The listing builds one solid part. Answer for the finished solid, in the listing's coordinates (mm). Face numbers are marked on the shaded views. A direction names the side the tool comes from. Give positions to 0.01 mm unless a question says otherwise; leave off trailing zeros. Write each loop counter-clockwise with the first axis right and the second up, starting at its lowest first coordinate (ties: lowest second). Pieces come first, ordered by that corner, then holes.
```python
from build123d import *

# Parameters (mm, degrees)
SKETCH1_W           = 122.77
SKETCH1_H           = 93
SKETCH1_R           = 1.63
BOSS_EXTRUDE1_DEPTH = 2
SKETCH2_W           = 2
SKETCH2_H           = 93
BOSS_EXTRUDE2_DEPTH = 31
SKETCH3_W           = 28.885
SKETCH3_H           = 73
SKETCH3_W_2         = 21
SKETCH3_H_2         = 83
CUT_EXTRUDE1_DEPTH  = 176.967075005


with BuildPart() as part:
    # Sketch1 → Boss-Extrude1 (new body)
    with BuildSketch(Plane(origin=(0, 0, 0), x_dir=(1, 0, 0), z_dir=(0, 1, 0))):
        with Locations((-105.371378726, 0.358527933)):
            Rectangle(SKETCH1_W, SKETCH1_H)
        with Locations(Location((-161.756378726, 41.858527933, 0), (0, 0, 270))):
            Circle(SKETCH1_R, mode=Mode.SUBTRACT)
        with Locations(Location((-48.986378726, 41.858527933, 0), (0, 0, 270))):
            Circle(SKETCH1_R, mode=Mode.SUBTRACT)
        with Locations(Location((-161.756378726, -41.141472067, 0), (0, 0, 270))):
            Circle(SKETCH1_R, mode=Mode.SUBTRACT)
        with Locations(Location((-48.986378726, -41.141472067, 0), (0, 0, 270))):
            Circle(SKETCH1_R, mode=Mode.SUBTRACT)
    extrude(amount=BOSS_EXTRUDE1_DEPTH)

    # Sketch2 → Boss-Extrude2 (add)
    with BuildSketch(Plane(origin=(0, 2, 0), x_dir=(1, 0, 0), z_dir=(0, 1, 0))):
        with Locations((-121.871378726, 0.358527933)):
            Rectangle(SKETCH2_W, SKETCH2_H)
        with Locations((-88.871378726, 0.358527933)):
            Rectangle(SKETCH2_W, SKETCH2_H)
    extrude(amount=BOSS_EXTRUDE2_DEPTH)

    # Sketch3 → Cut-Extrude1 (cut, through all)
    with BuildSketch(Plane(origin=(0, 2, 0), x_dir=(1, 0, 0), z_dir=(0, 1, 0))):
        with Locations((-142.313878726, 0.358527933)):
            Rectangle(SKETCH3_W, SKETCH3_H)
        with Locations((-105.371378726, 0.358527933)):
            Rectangle(SKETCH3_W_2, SKETCH3_H_2)
        with Locations((-68.428878726, 0.358527933)):
            Rectangle(SKETCH3_W, SKETCH3_H)
    extrude(amount=-CUT_EXTRUDE1_DEPTH, mode=Mode.SUBTRACT)


solid = part.part
```
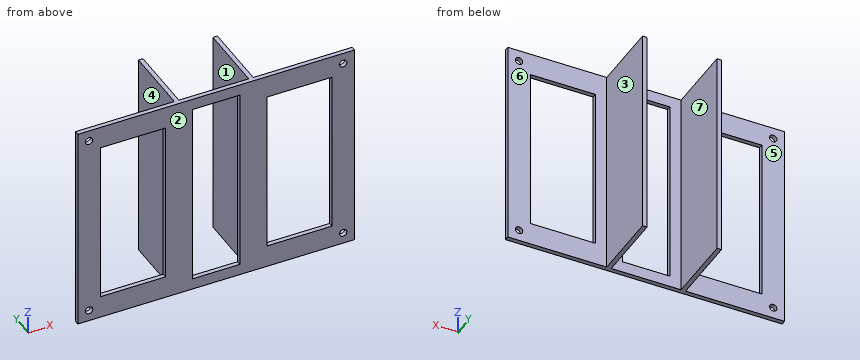
Item 1: A cutting plane is placed at B-B, the plane z = 38. Give the vertices of the cut face in (x, y), plus the area to 3 significant figures.
Conclusion:
outline: (-166.76, 0) - (-115.87, 0) - (-115.87, 2) - (-120.87, 2) - (-120.87, 33) - (-122.87, 33) - (-122.87, 2) - (-166.76, 2) - close; (-94.87, 0) - (-43.99, 0) - (-43.99, 2) - (-87.87, 2) - (-87.87, 33) - (-89.87, 33) - (-89.87, 2) - (-94.87, 2) - close
area: 328 mm2
Item 2: Which of the six approach directions +Z, -Z, +X, -X, +Y, -Y give full straight-line access (tool end or side, diameter ignored) to the marked faces 5, 6 and 7?
Conclusion:
face 5: +Z, -Z, -X, +Y
face 6: +Z, -Z, +X, +Y
face 7: +Z, -Z, +Y
Item 3: A cutting plane is placed at C-C, the plane y = 14.5. Give the vertices of the cut face in (x, z).
Conclusion:
outline: (-122.87, -46.86) - (-120.87, -46.86) - (-120.87, 46.14) - (-122.87, 46.14) - close; (-89.87, -46.86) - (-87.87, -46.86) - (-87.87, 46.14) - (-89.87, 46.14) - close
Item 4: Each of these flat-tipped pins is pushed along its axis until it touches: P1, Ø15.5, axis at y = 20, z = 7, coming from the -X side; P2, Ø1.5, axis at y = 7.5, z = -12, coming from the +X side; P3, Ø10, axis at x = -117.5, z = -30, coming from the -Y side; P4, Ø22, axis at x = -56.5, z = 14.5, coming from the +Y side. Where does it stop, or does it pass through?
Conclusion:
P1: stops at x = -122.87
P2: stops at x = -87.87
P3: stops at y = 0
P4: stops at y = 2
Item 5: A cutting plane is placed at A-A, the plane x = -62.5. Give the vertices of the cut face in (y, z).
Conclusion:
outline: (0, -46.86) - (2, -46.86) - (2, -36.86) - (0, -36.86) - close; (0, 36.14) - (2, 36.14) - (2, 46.14) - (0, 46.14) - close
Item 6: A cutting plane is placed at D-D, the plane z = -5. Give the vertices of the cut face in (x, y).
Conclusion:
outline: (-166.76, 0) - (-156.76, 0) - (-156.76, 2) - (-166.76, 2) - close; (-127.87, 0) - (-115.87, 0) - (-115.87, 2) - (-120.87, 2) - (-120.87, 33) - (-122.87, 33) - (-122.87, 2) - (-127.87, 2) - close; (-94.87, 0) - (-82.87, 0) - (-82.87, 2) - (-87.87, 2) - (-87.87, 33) - (-89.87, 33) - (-89.87, 2) - (-94.87, 2) - close; (-53.99, 0) - (-43.99, 0) - (-43.99, 2) - (-53.99, 2) - close
Item 7: Determine the mould class of the marked faces 1, 2, 3 and 4 for opening direction X: pulls with the +X half, pulls with the -X half, needs draft (parallel to the pull), parting line crosses it, or undercut.
Conclusion:
face 1: undercut
face 2: needs draft
face 3: pulls with the +X half
face 4: pulls with the -X half
Item 8: Consider probe 1 along X at (y, z) = (17, -15.5); probe 2 along Y at (x, z) = (-158, -36.5). Determine where each line is inside the solid, lowest interval first.
Conclusion:
probe 1: x = -122.87 to -120.87, -89.87 to -87.87
probe 2: y = 0 to 2
